Model file for the job. Use its own axes, mm. Face numbers are marked on the shaded views. A direction names the side the tool comes from. Round coordinates to 2 decimals unless told otherwise and drop trailing zeros. Order: outer loops, then holes, each group sorted by start corner. A loop starts at its lowest first (then second) coordinate and runs counter-clockwise, first axis right, second up. Notation, with made-up numbers: (49.5, 37.5) - (106.5, 37.5) arc R31 cw to (106.5, 72.5) - close; hole circle Ø4 at (-35, 30). An arc over 180 degrees is marked (long way). Write item = value, one per line.
```python
from build123d import *

# Parameters (mm, degrees)
BOSS_EXTRUDE1_DEPTH = 3
FILLET1_R           = 1
BOSS_EXTRUDE2_DEPTH = 18
BOSS_EXTRUDE2_DRAFT = -8
FILLET2_R           = 2
CUT_EXTRUDE1_DEPTH  = 61.545566409
FILLET4_R           = 10


with BuildPart() as part:
    # Sketch2 → Boss-Extrude1 (new body)
    with BuildSketch(Plane.XY):
        with BuildLine():
            Line((-5, -42.5), (5, -42.5))
            ThreePointArc((5, -42.5), (26.213203436, -33.713203436), (35, -12.5))
            Line((35, -12.5), (35, 12.5))
            ThreePointArc((35, 12.5), (26.213203436, 33.713203436), (5, 42.5))
            Line((5, 42.5), (-5, 42.5))
            ThreePointArc((-5, 42.5), (-26.213203436, 33.713203436), (-35, 12.5))
            Line((-35, 12.5), (-35, -12.5))
            ThreePointArc((-35, -12.5), (-26.213203436, -33.713203436), (-5, -42.5))
        make_face()
    extrude(amount=BOSS_EXTRUDE1_DEPTH)

    # Fillet1
    fillet1_edges = [part.edges().sort_by_distance(p)[0] for p in [
        (0, -42.5, 0),
        (-26.213203436, -33.713203436, 0),
        (-35, 0, 0),
        (-26.213203436, 33.713203436, 0),
        (-26.213203436, -33.713203436, 3),
        (0, -42.5, 3),
        (26.213203436, -33.713203436, 3),
        (35, 0, 3),
        (26.213203436, 33.713203436, 3),
        (0, 42.5, 3),
        (-26.213203436, 33.713203436, 3),
        (0, 42.5, 0),
        (-35, 0, 3),
        (26.213203436, 33.713203436, 0),
        (35, 0, 0),
        (26.213203436, -33.713203436, 0),
    ]]
    fillet(fillet1_edges, radius=FILLET1_R)


with BuildPart() as boss_extrude2_tool:
    # Sketch3 → Boss-Extrude2 (with draft: the straight prism first)
    with BuildSketch(Plane.XY.offset(3)):
        with BuildLine():
            Line((5, 41.5), (-5, 41.5))
            ThreePointArc((-5, 41.5), (-25.506096654, 33.006096654), (-34, 12.5))
            Line((-34, 12.5), (-34, -12.5))
            ThreePointArc((-34, -12.5), (-25.506096654, -33.006096654), (-5, -41.5))
            Line((-5, -41.5), (5, -41.5))
            ThreePointArc((5, -41.5), (25.506096654, -33.006096654), (34, -12.5))
            Line((34, -12.5), (34, 12.5))
            ThreePointArc((34, 12.5), (25.506096654, 33.006096654), (5, 41.5))
        make_face()
    extrude(amount=BOSS_EXTRUDE2_DEPTH)
    # Boss-Extrude2: the draft: its side faces are tilted about the plane it starts from
    boss_extrude2_sides = [boss_extrude2_tool.faces().sort_by_distance(p)[0] for p in [
        (-25.506096654, -33.006096654, 12),
        (0, -41.5, 12),
        (25.506096654, -33.006096654, 12),
        (34, 0, 12),
        (25.506096654, 33.006096654, 12),
        (0, 41.5, 12),
        (-25.506096654, 33.006096654, 12),
        (-34, 0, 12),
    ]]
    draft(boss_extrude2_sides, Plane.XY.offset(3), BOSS_EXTRUDE2_DRAFT)


with BuildPart() as part_1:
    add(part.part)

    # Boss-Extrude2: add boss_extrude2_tool
    add(boss_extrude2_tool.part)

    # Fillet2
    fillet2_edges = [part_1.edges().sort_by_distance(p)[0] for p in [
        (27.294889445, 34.794889445, 21),
        (0, 44.029735025, 21),
        (-27.294889445, 34.794889445, 21),
        (-36.529735025, 0, 21),
        (-27.294889445, -34.794889445, 21),
        (0, -44.029735025, 21),
        (27.294889445, -34.794889445, 21),
        (36.529735025, 0, 21),
    ]]
    fillet(fillet2_edges, radius=FILLET2_R)

    # Sketch5 → Cut-Extrude1 (cut, through all)
    with BuildSketch(Plane.XY.offset(21)):
        with BuildLine():
            Line((-10.75208941, -10), (-10.75208941, 10))
            ThreePointArc((-10.75208941, 10), (0, 20.75208941), (10.75208941, 10))
            Line((10.75208941, 10), (10.75208941, -10))
            ThreePointArc((10.75208941, -10), (0, -20.75208941), (-10.75208941, -10))
        make_face()
    extrude(amount=-CUT_EXTRUDE1_DEPTH, mode=Mode.SUBTRACT)

    # Fillet4
    fillet4_edges = [part_1.edges().sort_by_distance(p)[0] for p in [
        (0, -20.75208941, 0),
        (-10.75208941, 0, 0),
        (0, 20.75208941, 0),
        (10.75208941, 0, 0),
        (0, -20.75208941, 21),
        (10.75208941, 0, 21),
        (0, 20.75208941, 21),
        (-10.75208941, 0, 21),
    ]]
    fillet(fillet4_edges, radius=FILLET4_R)


solid = part_1.part
```
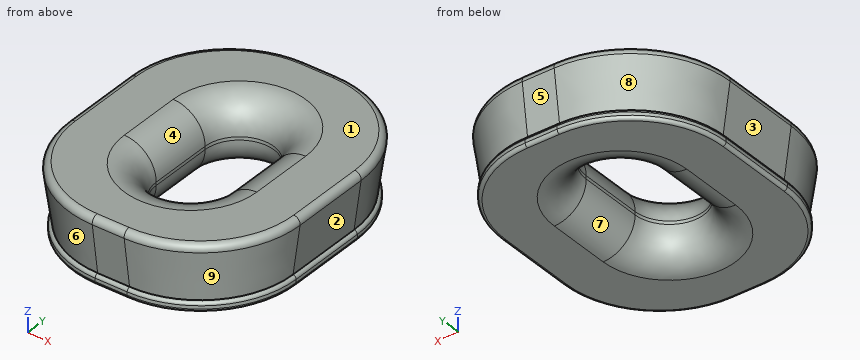
1) Cut at A-A (x = 0). Write the cut outline in (y, z), and give its area (3 significant figures).
Conclusion:
outline = (-43.71, 18.72) - (-41.5, 3) arc R1 ccw to (-42.5, 2) - (-42.5, 1) arc R1 ccw to (-41.5, 0) - (-30.75, 0) arc R10 ccw to (-20.75, 10) - (-20.75, 11) arc R10 ccw to (-30.75, 21) - (-41.73, 21) arc R2 ccw to start; (20.75, 10) arc R10 ccw to (30.75, 0) - (41.5, 0) arc R1 ccw to (42.5, 1) - (42.5, 2) arc R1 ccw to (41.5, 3) - (43.71, 18.72) arc R2 ccw to (41.73, 21) - (30.75, 21) arc R10 ccw to (20.75, 11) - close
area = 834 mm^2
2) Cut at C-C (z = 5.25). Write the cut outline in (x, y), and give its area (3 significant figures).
Conclusion:
outline = (-34.32, -12.5) arc R29.32 ccw to (-5, -41.82) - (5, -41.82) arc R29.32 ccw to (34.32, -12.5) - (34.32, 12.5) arc R29.32 ccw to (5, 41.82) - (-5, 41.82) arc R29.32 ccw to (-34.32, 12.5) - close; hole (-11.95, -10) arc R11.95 ccw to (11.95, -10) - (11.95, 10) arc R11.95 ccw to (-11.95, 10) - close
area = 4,080 mm^2
3) Wall check: line 1 along Y through (x, z) = (-0.5, 8.5); line 2 along X through (y, z) = (19.5, 8.5); line 3 along Y through (x, z) = (8.5, 11.25). Give the ranges that are in metal, low to high.
Conclusion:
line_1 = -42.27 to -20.85, 20.85 to 42.27
line_2 = -33.94 to -5.27, 5.27 to 33.94
line_3 = -42.46 to -16.59, 16.59 to 42.46
4) Cut at B-B (y = 3). Write the cut outline in (x, z).
Conclusion:
outline = (-36.21, 18.72) - (-34, 3) arc R1 ccw to (-35, 2) - (-35, 1) arc R1 ccw to (-34, 0) - (-20.75, 0) arc R10 ccw to (-10.75, 10) - (-10.75, 11) arc R10 ccw to (-20.75, 21) - (-34.23, 21) arc R2 ccw to start; (10.75, 10) arc R10 ccw to (20.75, 0) - (34, 0) arc R1 ccw to (35, 1) - (35, 2) arc R1 ccw to (34, 3) - (36.21, 18.72) arc R2 ccw to (34.23, 21) - (20.75, 21) arc R10 ccw to (10.75, 11) - close
5) Flat gauge pins, fed straight in: pin 1 Ø0.5 at (y, z) = (0, 1.5) entering from -X; pin 2 Ø1.1 at (x, z) = (-0.5, 1.5) entering from +Y; pin 3 Ø1 at (y, z) = (-24.5, 16) entering from +X. Where does each tip first touch, or does it go through?
Conclusion:
pin_1 = -35
pin_2 = 42.5
pin_3 = 33.62
6) 3-axis set-ups, long thin cutter, end or side, ignore diameter. For the marked faces 5, 6, 7, 8 and 9: which of +Z, -Z, +X, -X, +Y, -Y reach the whole face in a straight line?
Conclusion:
face_5 = +X, -X, +Y
face_6 = -X, -Y
face_7 = -Z
face_8 = -X, +Y
face_9 = +X, -Y
7) Mould opens along X. For the marked faces 1, 2, 3 and 4 say: +X half, -X half, draft (parallel to the pull), parting line (faces both ways), or undercut.
Conclusion:
face_1 = draft
face_2 = +X half
face_3 = -X half
face_4 = undercut
